Could you check a few things on this model? Use its own coordinates, in mm. Face numbers are marked on the shaded views. A direction names the side the tool comes from. Coordinates: 2 decimals unless noted, no trailing zeros. Write each loop counter-clockwise with the first axis right and the second up, starting at its lowest first coordinate (ties: lowest second). Pieces come first, ordered by that corner, then holes. Notation, with made-up numbers: (-6, 9.5) - (36, 9.5) arc R29 cw to (36, 38.5) - close; hole circle Ø10 at (78, -17.5). An arc over 180 degrees is marked (long way). Answer as a JSON object with one key per item and string values. Group by question number.
1) If we section it at D-D (x = 25): Write out the boundary of the cut face in (y, z).
2) Will these pins go through, and if not, where does the flat tip stop? pin 1 Ø1.5 at (x, z) = (0.5, -25.5) entering from -Y; pin 2 Ø4 at (x, z) = (-25, 0) entering from +Y; pin 3 Ø1 at (x, y) = (1, 17) entering from -Z.
3) Please list where these lines run through material, in increasing order: line 1 along Y through (x, z) = (-6, 29); line 2 along Z through (x, y) = (3, 3); line 3 along Y through (x, z) = (-22, -10).
4) On a 3-axis mill with a long thin cutter (end or side, diameter ignored), from which of +Z, -Z, +X, -X, +Y, -Y can I reach the whole of each face in a straight line? I mean the marked faces 1 and 2. Say none if no direction works.
5) If we section it at C-C (y = -3): Write out the boundary of the cut face in (x, z).
6) We'd pull the mould along Z, two halves only. Please class the marked faces 3, 4 and 5: released by +Z, released by -Z, zero draft, split by the parting line, or undercut.
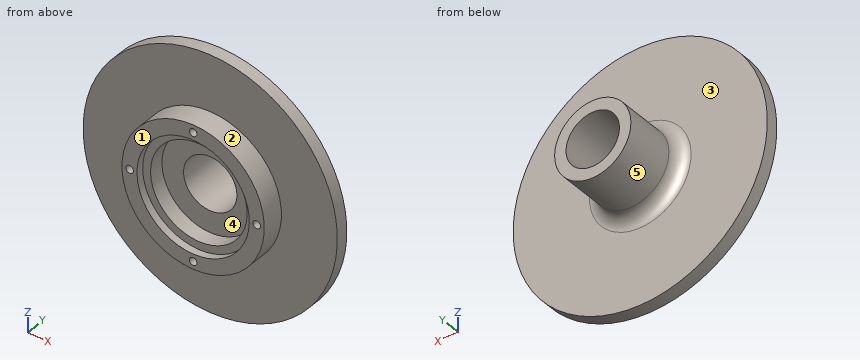
```python
from build123d import *

# Parameters (mm, degrees)
SKETCH_1_R          = 50
SKETCH_1_R_2        = 10.5
EXTRUDE_1_DEPTH     = 30
SKETCH_2_R          = 54.511418905
SKETCH_2_R_2        = 15
CUT_EXTRUDE_2_DEPTH = 25
SKETCH_3_R          = 28
SKETCH_3_R_2        = 19
SKETCH_3_R_3        = 1.5
EXTRUDE_3_DEPTH     = 9
SKETCH_4_R          = 22.1
CUT_EXTRUDE_4_DEPTH = 3
FILLET_3_R          = 5


with BuildPart() as part:
    # Эскиз1 → Вытянуть1 (new body)
    with BuildSketch(Plane(origin=(0, 0, 0), x_dir=(1, 0, 0), z_dir=(0, 1, 0))):
        with Locations(Location((0, 0, 0), (0, 0, 270))):
            Circle(SKETCH_1_R)
        with Locations(Location((0, 0, 0), (0, 0, 270))):
            Circle(SKETCH_1_R_2, mode=Mode.SUBTRACT)
    extrude(amount=EXTRUDE_1_DEPTH)

    # Эскиз2 → Вытянуть2 (cut)
    with BuildSketch(Plane(origin=(0, 30, 0), x_dir=(1, 0, 0), z_dir=(0, 1, 0))):
        Circle(SKETCH_2_R)
        with Locations(Location((0, 0, 0), (0, 0, 270))):
            Circle(SKETCH_2_R_2, mode=Mode.SUBTRACT)
    extrude(amount=-CUT_EXTRUDE_2_DEPTH, mode=Mode.SUBTRACT)

    # Эскиз3 → Вытянуть3 (add)
    with BuildSketch(Plane.XZ):
        with Locations(Location((0, 0, 0), (0, 0, 90))):
            Circle(SKETCH_3_R)
        with Locations(Location((0, 0, 0), (0, 0, 270))):
            Circle(SKETCH_3_R_2, mode=Mode.SUBTRACT)
        with Locations(Location((0, 25, 0), (0, 0, 270))):
            Circle(SKETCH_3_R_3, mode=Mode.SUBTRACT)
        with Locations(Location((25, 0, 0), (0, 0, 270))):
            Circle(SKETCH_3_R_3, mode=Mode.SUBTRACT)
        with Locations(Location((0, -25, 0), (0, 0, 270))):
            Circle(SKETCH_3_R_3, mode=Mode.SUBTRACT)
        with Locations(Location((-25, 0, 0), (0, 0, 270))):
            Circle(SKETCH_3_R_3, mode=Mode.SUBTRACT)
    extrude(amount=EXTRUDE_3_DEPTH)

    # Эскиз4 → Вытянуть4 (cut)
    with BuildSketch(Plane.XZ.offset(9)):
        with Locations(Location((0, 0, 0), (0, 0, 270))):
            Circle(SKETCH_4_R)
    extrude(amount=-CUT_EXTRUDE_4_DEPTH, mode=Mode.SUBTRACT)

    # Скругление3
    fillet_3_edges = [part.edges().sort_by_distance(p)[0] for p in [
        (0, 5, -15),
    ]]
    fillet(fillet_3_edges, radius=FILLET_3_R)


solid = part.part
```
Here are the results:
{
 "1": {"outline": "(-9, -12.61) - (0, -12.61) - (0, -43.3) - (5, -43.3) - (5, 43.3) - (0, 43.3) - (0, 12.61) - (-9, 12.61) - (-9, 1.5) - (0, 1.5) - (0, -1.5) - (-9, -1.5) - close"},
 "2": {"pin 1": "stops at y = 0", "pin 2": "stops at y = 5", "pin 3": "stops at z = -14.99"},
 "3": {"line 1": "y = 0 to 5", "line 2": "z = -49.91 to -10.06, 10.06 to 49.91", "line 3": "y = -9 to 5"},
 "4": {"face 1": "+Z, -Z, +X, -X, -Y", "face 2": "-Y"},
 "5": {"outline": "circle Ø56 at (0, 0); hole circle Ø3 at (-25, 0); hole circle Ø38 at (0, 0); hole circle Ø3 at (0, -25); hole circle Ø3 at (0, 25); hole circle Ø3 at (25, 0)"},
 "6": {"face 3": "zero draft", "face 4": "undercut", "face 5": "split by the parting line"}
}
